from build123d import *

# Parameters (mm, degrees)
F1_DEPTH = 76.2
F2_W     = 153.924
F2_H     = 153.924
F3_DEPTH = 3.175
F4_W     = 149.86
F4_H     = 149.86
F5_DEPTH = 63.5


# Not quite as in the source:
# - a feature names something its author has since deleted; it is built from what else it names


with BuildPart() as f1:
    # F0 (on Front) → F1 (new body)
    with BuildSketch(Plane.XZ):
        Polygon((0, 139.7), (0, 158.75), (-158.75, 158.75), (-158.75, 0), (-139.7, 0), (-139.7, 139.7), align=None)
    extrude(amount=F1_DEPTH)

    # F2 (on face) → F3 (cut)
    with BuildSketch(Plane.XZ.offset(76.2)):
        with Locations((-76.962, 76.962)):
            Rectangle(F2_W, F2_H)
    extrude(amount=-F3_DEPTH, mode=Mode.SUBTRACT)

    # F4 (on face) → F5 (cut)
    with BuildSketch(Plane.XZ.offset(73.025)):
        with Locations((-74.93, 74.93)):
            Rectangle(F4_W, F4_H)
    extrude(amount=-F5_DEPTH, mode=Mode.SUBTRACT)


solid = f1.part
Input: part model. Units: mm. Frame: model coordinates. A direction names the side the tool comes from. Give positions to 0.01 mm unless a question says otherwise; leave off trailing zeros. Order: outer loops, then holes, each group sorted by start corner. A loop starts at its lowest first (then second) coordinate and runs counter-clockwise, first axis right, second up.
Q1. Section A-A on z = 84. Output: boundary loops of the cut face in (x, y) (3 decimals), and give its area (3 significant figures).
Checked values:
outline: (-158.75, -76.2) - (-153.924, -76.2) - (-153.924, -73.025) - (-149.86, -73.025) - (-149.86, -9.525) - (-139.7, -9.525) - (-139.7, 0) - (-158.75, 0) - close
area: 761 mm2
Q2. Ray query, probe 1 along Z at (x, y) = (-37, -62); probe 2 along Y at (x, z) = (-149, 150.5) (3 decimals); probe 3 along X at (y, z) = (-69.5, 133). Return the intervals inside material, ascending.
Checked values:
probe 1: z = 149.86 to 158.75
probe 2: y = -73.025 to 0
probe 3: x = -158.75 to -149.86
Q3. Set-up query: faces 1 (the flat face through (-154, -38, 0)), 2 (the flat face through (-71, -5, 139.7)), 3 (the flat face through (-151, -73.025, 112)). Return all of +Z, -Z, +X, -X, +Y, -Y with unobstructed straight access to the full face (end or side cutting, diameter ignored); none if empty.
Checked values:
face 1: -Z, +X, -X, +Y, -Y
face 2: -Z, +X, +Y, -Y
face 3: -Z, +X, -Y
Q4. Contact query for flat-ended pins moving along their axis: pin 1 Ø2 at (y, z) = (-26, 137.5) entering from +X; pin 2 Ø2 at (x, y) = (-70, -39.5) entering from -Z; pin 3 Ø3 at (x, y) = (-87, -2.5) entering from -Z. Output: stop coordinate, or through.
Checked values:
pin 1: stops at x = -149.86
pin 2: stops at z = 149.86
pin 3: stops at z = 139.7
Q5. Section B-B on x = -43. Output: boundary loops of the cut face in (y, z) (3 decimals), and give its area (3 significant figures).
Checked values:
outline: (-76.2, 153.924) - (-73.025, 153.924) - (-73.025, 149.86) - (-9.525, 149.86) - (-9.525, 139.7) - (0, 139.7) - (0, 158.75) - (-76.2, 158.75) - close
area: 761 mm2
Q6. Section C-C on y = -37.5. Output: boundary loops of the cut face in (x, z).
Checked values:
outline: (-158.75, 0) - (-149.86, 0) - (-149.86, 149.86) - (0, 149.86) - (0, 158.75) - (-158.75, 158.75) - close
